Work out the finished part from the listing and answer in its coordinate system (mm). Face numbers are marked on the shaded views. Round coordinates to 2 decimals unless told otherwise and drop trailing zeros. Order: outer loops, then holes, each group sorted by start corner. A loop starts at its lowest first (then second) coordinate and runs counter-clockwise, first axis right, second up. Notation, with made-up numbers: (66.5, 13.5) -> (124.5, 13.5) arc R32 ccw to (124.5, 40.5) -> close; hole circle Ø8 at (24.25, 89.25). An arc over 180 degrees is marked (long way). Use one line per item in the form item = value.
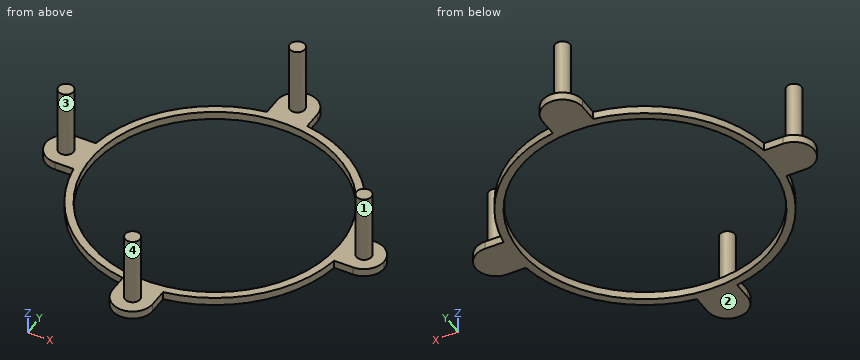
```python
from build123d import *

# Parameters (mm, degrees)
F0_R     = 30.75
F0_R_2   = 1.85
F1_DEPTH = 2
F2_DEPTH = 19


with BuildPart() as f1:
    # F0 (on Top) → F1 (new body)
    with BuildSketch(Plane.XY):
        with BuildLine():
            ThreePointArc((32.65625, 2.476254417), (32.5356397493, 3.7409418742), (32.366070197, 5))
            ThreePointArc((32.366070197, 5), (23.1577470839, 23.1577470839), (5, 32.366070197))
            ThreePointArc((5, 32.366070197), (3.7409418742, 32.5356397493), (2.476254417, 32.65625))
            ThreePointArc((2.476254417, 32.65625), (0, 32), (-2.476254417, 32.65625))
            ThreePointArc((-2.476254417, 32.65625), (-3.7409418742, 32.5356397493), (-5, 32.366070197))
            ThreePointArc((-5, 32.366070197), (-23.1577470839, 23.1577470839), (-32.366070197, 5))
            ThreePointArc((-32.366070197, 5), (-32.5356397493, 3.7409418742), (-32.65625, 2.476254417))
            ThreePointArc((-32.65625, 2.476254417), (-32.1668462677, 1.2808688457), (-32, 0))
            ThreePointArc((-32, 0), (-32.1668462677, -1.2808688457), (-32.65625, -2.476254417))
            ThreePointArc((-32.65625, -2.476254417), (-32.5356397493, -3.7409418742), (-32.366070197, -5))
            ThreePointArc((-32.366070197, -5), (-23.1577470839, -23.1577470839), (-5, -32.366070197))
            ThreePointArc((-5, -32.366070197), (-3.7409418742, -32.5356397493), (-2.476254417, -32.65625))
            ThreePointArc((-2.476254417, -32.65625), (0, -32), (2.476254417, -32.65625))
            ThreePointArc((2.476254417, -32.65625), (3.7409418742, -32.5356397493), (5, -32.366070197))
            ThreePointArc((5, -32.366070197), (23.1577470839, -23.1577470839), (32.366070197, -5))
            ThreePointArc((32.366070197, -5), (32.5356397493, -3.7409418742), (32.65625, -2.476254417))
            ThreePointArc((32.65625, -2.476254417), (32, 0), (32.65625, 2.476254417))
        make_face()
        Circle(F0_R, mode=Mode.SUBTRACT)
        with BuildLine():
            Line((37, 5), (32.366070197, 5))
            ThreePointArc((32.366070197, 5), (32.5356397493, 3.7409418742), (32.65625, 2.476254417))
            ThreePointArc((32.65625, 2.476254417), (34.488155268, 4.3232668253), (37, 5))
        make_face()
        with BuildLine():
            ThreePointArc((2.476254417, 32.65625), (3.7409418742, 32.5356397493), (5, 32.366070197))
            Line((5, 32.366070197), (5, 37))
            ThreePointArc((5, 37), (4.3232668253, 34.488155268), (2.476254417, 32.65625))
        make_face()
        with BuildLine():
            ThreePointArc((37, 5), (34.488155268, 4.3232668253), (32.65625, 2.476254417))
            ThreePointArc((32.65625, 2.476254417), (32.7265541075, 1.2390142251), (32.75, 0))
            ThreePointArc((32.75, 0), (32.7265541075, -1.2390142251), (32.65625, -2.476254417))
            ThreePointArc((32.65625, -2.476254417), (34.488155268, -4.3232668253), (37, -5))
            ThreePointArc((37, -5), (40.5355339059, -3.5355339059), (42, 0))
            ThreePointArc((42, 0), (40.5355339059, 3.5355339059), (37, 5))
        make_face()
        with Locations((37, 0)):
            Circle(F0_R_2, mode=Mode.SUBTRACT)
        with BuildLine():
            ThreePointArc((-2.476254417, 32.65625), (0, 32.75), (2.476254417, 32.65625))
            ThreePointArc((2.476254417, 32.65625), (4.3232668253, 34.488155268), (5, 37))
            ThreePointArc((5, 37), (0, 42), (-5, 37))
            ThreePointArc((-5, 37), (-4.3232668253, 34.488155268), (-2.476254417, 32.65625))
        make_face()
        with Locations((0, 37)):
            Circle(F0_R_2, mode=Mode.SUBTRACT)
        with BuildLine():
            ThreePointArc((37, -5), (34.488155268, -4.3232668253), (32.65625, -2.476254417))
            ThreePointArc((32.65625, -2.476254417), (32.5356397493, -3.7409418742), (32.366070197, -5))
            Line((32.366070197, -5), (37, -5))
        make_face()
        with BuildLine():
            ThreePointArc((-5, 32.366070197), (-3.7409418742, 32.5356397493), (-2.476254417, 32.65625))
            ThreePointArc((-2.476254417, 32.65625), (-4.3232668253, 34.488155268), (-5, 37))
            Line((-5, 37), (-5, 32.366070197))
        make_face()
        with BuildLine():
            Line((5, -37), (5, -32.366070197))
            ThreePointArc((5, -32.366070197), (3.7409418742, -32.5356397493), (2.476254417, -32.65625))
            ThreePointArc((2.476254417, -32.65625), (4.3232668253, -34.488155268), (5, -37))
        make_face()
        with BuildLine():
            ThreePointArc((-32.65625, 2.476254417), (-32.5356397493, 3.7409418742), (-32.366070197, 5))
            Line((-32.366070197, 5), (-37, 5))
            ThreePointArc((-37, 5), (-34.488155268, 4.3232668253), (-32.65625, 2.476254417))
        make_face()
        with BuildLine():
            ThreePointArc((5, -37), (4.3232668253, -34.488155268), (2.476254417, -32.65625))
            ThreePointArc((2.476254417, -32.65625), (0, -32.75), (-2.476254417, -32.65625))
            ThreePointArc((-2.476254417, -32.65625), (-4.3232668253, -34.488155268), (-5, -37))
            ThreePointArc((-5, -37), (0, -42), (5, -37))
        make_face()
        with Locations((0, -37)):
            Circle(F0_R_2, mode=Mode.SUBTRACT)
        with BuildLine():
            ThreePointArc((-32.65625, -2.476254417), (-32.75, 0), (-32.65625, 2.476254417))
            ThreePointArc((-32.65625, 2.476254417), (-34.488155268, 4.3232668253), (-37, 5))
            ThreePointArc((-37, 5), (-42, 0), (-37, -5))
            ThreePointArc((-37, -5), (-34.488155268, -4.3232668253), (-32.65625, -2.476254417))
        make_face()
        with Locations((-37, 0)):
            Circle(F0_R_2, mode=Mode.SUBTRACT)
        with BuildLine():
            ThreePointArc((-5, -37), (-4.3232668253, -34.488155268), (-2.476254417, -32.65625))
            ThreePointArc((-2.476254417, -32.65625), (-3.7409418742, -32.5356397493), (-5, -32.366070197))
            Line((-5, -32.366070197), (-5, -37))
        make_face()
        with BuildLine():
            ThreePointArc((-32.366070197, -5), (-32.5356397493, -3.7409418742), (-32.65625, -2.476254417))
            ThreePointArc((-32.65625, -2.476254417), (-34.488155268, -4.3232668253), (-37, -5))
            Line((-37, -5), (-32.366070197, -5))
        make_face()
        with BuildLine():
            ThreePointArc((-2.476254417, 32.65625), (0, 32), (2.476254417, 32.65625))
            ThreePointArc((2.476254417, 32.65625), (0, 32.75), (-2.476254417, 32.65625))
        make_face()
        with BuildLine():
            ThreePointArc((-32, 0), (-32.1668462677, 1.2808688457), (-32.65625, 2.476254417))
            ThreePointArc((-32.65625, 2.476254417), (-32.75, 0), (-32.65625, -2.476254417))
            ThreePointArc((-32.65625, -2.476254417), (-32.1668462677, -1.2808688457), (-32, 0))
        make_face()
        with BuildLine():
            ThreePointArc((-2.476254417, -32.65625), (0, -32.75), (2.476254417, -32.65625))
            ThreePointArc((2.476254417, -32.65625), (0, -32), (-2.476254417, -32.65625))
        make_face()
        with BuildLine():
            ThreePointArc((32.75, 0), (32.7265541075, 1.2390142251), (32.65625, 2.476254417))
            ThreePointArc((32.65625, 2.476254417), (32, 0), (32.65625, -2.476254417))
            ThreePointArc((32.65625, -2.476254417), (32.7265541075, -1.2390142251), (32.75, 0))
        make_face()
    extrude(amount=F1_DEPTH)

    # F0 (on Top) → F2 (join)
    with BuildSketch(Plane.XY):
        with Locations((0, 37)):
            Circle(F0_R_2)
        with Locations((-37, 0)):
            Circle(F0_R_2)
        with Locations((0, -37)):
            Circle(F0_R_2)
        with Locations((37, 0)):
            Circle(F0_R_2)
    extrude(amount=F2_DEPTH)


solid = f1.part
```
Item 1: The part is cut by section C-C, the plane z = 12. Give the vertices of the cut face in (x, y).
Findings:
outline = circle Ø3.7 at (-37, 0); circle Ø3.7 at (0, -37); circle Ø3.7 at (0, 37); circle Ø3.7 at (37, 0)
Item 2: The part is cut by section A-A, the plane x = 0. Give the vertices of the cut face in (y, z).
Findings:
outline = (-42, 0) -> (-30.75, 0) -> (-30.75, 2) -> (-35.15, 2) -> (-35.15, 19) -> (-38.85, 19) -> (-38.85, 2) -> (-42, 2) -> close; (30.75, 0) -> (42, 0) -> (42, 2) -> (38.85, 2) -> (38.85, 19) -> (35.15, 19) -> (35.15, 2) -> (30.75, 2) -> close
Item 3: Determine the mould class of the marked faces 1, 2, 3 and 4 for opening direction X: released by +X, released by -X, zero draft, split by the parting line, or undercut.
Findings:
face_1 = undercut
face_2 = zero draft
face_3 = undercut
face_4 = split by the parting line
Item 4: The part is cut by section B-B, the plane y = 16.5. Give the vertices of the cut face in (x, z), and give its area (3 significant figures).
Findings:
outline = (-28.29, 0) -> (-25.95, 0) -> (-25.95, 2) -> (-28.29, 2) -> close; (25.95, 0) -> (28.29, 0) -> (28.29, 2) -> (25.95, 2) -> close
area = 9.37 mm^2
Item 5: Flat-ended cylindrical pins translate along their axes: P1, Ø1, axis at x = 35.5, z = 1.5, coming from the -Y side; P2, Ø2, axis at x = 34, z = 1, coming from the +Y side; P3, Ø1.6, axis at y = -34, z = 1, coming from the -X side. Find the tip coordinate at first contact, or state that the pin passes through.
Findings:
P1 = -5
P2 = 5
P3 = -5
Item 6: The part is cut by section D-D, the plane x = -20. Give the vertices of the cut face in (y, z), and give its area (3 significant figures).
Findings:
outline = (-25.93, 0) -> (-23.36, 0) -> (-23.36, 2) -> (-25.93, 2) -> close; (23.36, 0) -> (25.93, 0) -> (25.93, 2) -> (23.36, 2) -> close
area = 10.3 mm^2
Item 7: Consider line 1 along Y through (x, z) = (0, 0.7); line 2 along Y through (x, z) = (0, 9); line 3 along X through (y, z) = (-26.5, 1.25). Determine where each line is inside the solid, lowest interval first.
Findings:
line_1 = -42 to -30.75, 30.75 to 42
line_2 = -38.85 to -35.15, 35.15 to 38.85
line_3 = -19.24 to -15.6, 15.6 to 19.24
